Autodesk Inventor part; units mm, degrees
ref_plane "YZ Plane" through (0, 0, 0) normal (1, 0, 0) x (0, 1, 0)
ref_plane "XZ Plane" through (0, 0, 0) normal (0, 1, 0) x (-1, 0, 0)
ref_plane "XY Plane" through (0, 0, 0) normal (0, 0, 1) x (1, 0, 0)
sketch "Sketch1" plane through (0, 0, 0) normal (0, 1, 0) x (-1, 0, 0)
  line L0 (-5, 5) -> (5, 5)
  line L1 (5, 5) -> (5, -5)
  line L2 (5, -5) -> (-5, -5)
  line L3 (-5, -5) -> (-5, 5)
  line L4 (-5, 5) -> (5, -5) construction
  line L5 (5, 5) -> (-5, -5) construction
  point P0 (0, 0)
  dimension "d0" = 10
  dimension "d1" = 10
extrude "Extrusion1" add sketch "Sketch1" along normal blind 1.5
sketch "Sketch3" plane through (0, 1.5, 0) normal (0, 1, 0) x (1, 0, 0)
  line L0 (-5, -5) -> (-5, 5)
  line L1 (-5, 5) -> (-3.5, 5)
  line L2 (5, 5) -> (-5, 5)
  line L3 (-3.5, 5) -> (-3.5, -3.5)
  line L4 (-3.5, -3.5) -> (5, -3.5)
  line L5 (5, -3.5) -> (5, -5)
  line L6 (5, -5) -> (-5, -5)
  point P0 (0, 0)
  dimension "d7" = 1.5
  dimension "d8" = 8.5
  dimension "d9" = 90
extrude "Extrusion2" add sketch "Sketch3" along normal blind 8.5
sketch "Sketch5" plane through (0, 1.5, 0) normal (0, 1, 0) x (1, 0, 0)
  circle A0 centre (-2.5, 0.8) radius 0.5
  line L0 (-3.5, 5) -> (-3.5, -3.5)
  line L1 (-3.5, -3.5) -> (5, -3.5)
  point P0 (0, 0)
  dimension "d14" = 1
  dimension "d15" = 1
  dimension "d16" = 4.3
extrude "Extrusion4" cut sketch "Sketch5" against normal blind 8.5
sketch "Sketch6" plane through (-3.5, 1.5, 3.5) normal (1, 0, 0) x (0, 0, -1)
  circle A0 centre (1, 4.3) radius 0.5
  line L0 (8.5, 0) -> (0, 0)
  line L1 (0, 0) -> (0, 8.5)
  point P0 (3.5, -1.5)
  point P1 (0, 7)
  dimension "d19" = 1
  dimension "d20" = 4.3
  dimension "d21" = 1
extrude "Extrusion5" cut sketch "Sketch6" against normal blind 8.5
sketch "Sketch7" plane through (5, 1.5, 3.5) normal (0, 0, -1) x (-1, 0, 0)
  circle A0 centre (4.2, 1) radius 0.5
  line L0 (8.5, 0) -> (0, 0)
  line L1 (8.5, 0) -> (8.5, 8.5)
  point P0 (5, -1.5)
  dimension "d24" = 1
  dimension "d25" = 1
  dimension "d26" = 4.3
extrude "Extrusion6" cut sketch "Sketch7" against normal blind 8.5
sketch "Sketch8" plane through (0, 10, 0) normal (0, 1, 0) x (1, 0, 0)
  line L0 (5, -5) -> (5, 5)
  line L1 (5, 5) -> (-5, 5)
  line L2 (-5, 5) -> (-5, -5)
  line L3 (-5, -5) -> (5, -5)
  point P0 (0, 0)
extrude "Extrusion7" add sketch "Sketch8" along normal blind 1.5
sketch "Sketch9" plane through (0, 11.5, 0) normal (0, 1, 0) x (1, 0, 0)
  circle A0 centre (1, 1) radius 1
  line L0 (-5, 5) -> (-5, -5)
  line L1 (-5, -5) -> (5, -5)
  point P0 (0, 0)
  dimension "d31" = 2
  dimension "d32" = 6
  dimension "d33" = 6
extrude "Extrusion8" cut sketch "Sketch9" against normal blind 1.5
properties part number "Corner"
The model under review builds one solid part; all positions refer to its coordinate system, in mm. A direction names the side the tool comes from. Give positions to 0.01 mm unless a question says otherwise; leave off trailing zeros. Loops run counter-clockwise (first coordinate to the right, second up) from the corner with the lowest first, then second, coordinate; pieces in that order, holes last. Notation, with made-up numbers: (20, 58.25) -> (58, 58.25) arc R29 cw to (58, 88.25) -> close; hole circle Ø1 at (71, 42.5). An arc over 180 degrees is marked (long way). Write each question's results on one line, items separated by ' | '.
1) For line 1 along Y through (x, z) = (-4.55, 2.5); line 2 along Z through (x, y) = (-2.5, 1.2); line 3 along X through (y, z) = (0.65, -0.8), list the stretches that pass through material, from the lowest coordinate up. Write a range as from..to.
Conclusion:
line 1: y = 0..5.3, 6.3..11.5 | line 2: z = -5..-1.3, -0.3..5 | line 3: x = -5..-3, -2..5
2) Take a section at A-A, the plane y = 2.5. Give the boundary of the cut face in (x, z), plus the area to 4 significant figures.
Conclusion:
outline: (-5, -5) -> (-3.5, -5) -> (-3.5, 3.5) -> (0.3, 3.5) -> (0.3, 5) -> (-5, 5) -> close; (1.3, 3.5) -> (5, 3.5) -> (5, 5) -> (1.3, 5) -> close | area: 26.25 mm^2
3) Insertion check: pin 1 Ø4 at (y, z) = (7, 0.5) entering from +X; pin 2 Ø1.2 at (x, z) = (1, -1) entering from +Y; pin 3 Ø4 at (x, y) = (0.5, 6) entering from -Z. Each pin has a flat end and moves straight along its axis. Give the tip position at first contact, or say it passes through.
Conclusion:
pin 1: stops at x = -3.5 | pin 2: stops at y = 1.5 | pin 3: stops at z = 3.5
4) Take a section at C-C, the plane z = -1.75. Give the boundary of the cut face in (x, y).
Conclusion:
outline: (-5, 0) -> (5, 0) -> (5, 1.5) -> (-3.5, 1.5) -> (-3.5, 10) -> (0.34, 10) -> (0.34, 11.5) -> (-5, 11.5) -> close; (1.66, 10) -> (5, 10) -> (5, 11.5) -> (1.66, 11.5) -> close
5) Draft analysis for pull direction Z (two halves, no side actions). For faces 4 (the face through (-2.9, 0.8, -0.5)), 5 (the face through (0.5, 2.9, 4.2)), 6 (the face through (1, 6, 3.5)), state which applies: pulls with the +Z half, pulls with the -Z half, needs draft (parallel to the pull), parting line crosses it, or undercut.
Conclusion:
face 4: undercut | face 5: needs draft | face 6: pulls with the -Z half
6) Tool access review of faces 1 (the face through (-3.5, 6, -1)), 2 (the face through (1, 11, 0)), 3 (the face through (0, 6, 5)): name each direction out of +Z, -Z, +X, -X, +Y, -Y from which nothing blocks a thin tool from reaching the whole face with its end or side.
Conclusion:
face 1: -Z, +X | face 2: +Y | face 3: +Z, +X, -X, +Y, -Y
7) Take a section at D-D, the plane x = 1. Give the boundary of the cut face in (y, z).
Conclusion:
outline: (0, -5) -> (1.5, -5) -> (1.5, 3.5) -> (2.04, 3.5) -> (2.04, 5) -> (0, 5) -> close; (2.96, 3.5) -> (10, 3.5) -> (10, 0) -> (11.5, 0) -> (11.5, 5) -> (2.96, 5) -> close; (10, -5) -> (11.5, -5) -> (11.5, -2) -> (10, -2) -> close
8) Take a section at B-B, the plane x = -2.5. Give the boundary of the cut face in (y, z).
Conclusion:
outline: (0, -5) -> (1.5, -5) -> (1.5, -1.3) -> (0, -1.3) -> close; (0, -0.3) -> (1.5, -0.3) -> (1.5, 3.5) -> (10, 3.5) -> (10, -5) -> (11.5, -5) -> (11.5, 5) -> (0, 5) -> close
